The model under review builds one solid part; all positions refer to its coordinate system, in mm. A direction names the side the tool comes from. Round coordinates to 2 decimals unless told otherwise and drop trailing zeros. Order: outer loops, then holes, each group sorted by start corner. A loop starts at its lowest first (then second) coordinate and runs counter-clockwise, first axis right, second up. Notation, with made-up numbers: M -24,33 L 20,33 A35 ccw 20,72 Z; hole C 88.5,1.5 d5. An arc over 180 degrees is marked long. Answer as CSV lines item,"result". Start each with the question number.
from build123d import *

# Parameters (mm, degrees)
SKETCH1_R           = 1.525
SKETCH1_W           = 3
SKETCH1_H           = 19.5
BOSS_EXTRUDE1_DEPTH = 5
FILLET4_R           = 3
FILLET5_R           = 1
SKETCH4_R           = 3
CUT_EXTRUDE1_DEPTH  = 3
FILLET6_R           = 8
SKETCH6_R           = 19.727216355
CUT_EXTRUDE2_DEPTH  = 6
SKETCH9_R           = 9
CUT_EXTRUDE3_DEPTH  = 8.5
SKETCH11_W          = 2
SKETCH11_H          = 5
SKETCH11_W_2        = 10
SKETCH11_H_2        = 3
CUT_EXTRUDE4_DEPTH  = 6
FILLET7_R           = 1
SKETCH13_R          = 1.525
SKETCH13_W          = 3.25
SKETCH13_H          = 9
CUT_EXTRUDE5_DEPTH  = 6
FILLET8_R           = 1


with BuildPart() as part:
    # Sketch1 → Boss-Extrude1 (new body)
    with BuildSketch(Plane(origin=(0, 0, 0), x_dir=(1, 0, 0), z_dir=(0, 1, 0))):
        Polygon((-26.68337521, 71.16), (-26.68337521, 34), (-32.68337521, 28), (-20.1, 28), (-20.1, -28), (-32.68337521, -28), (-26.68337521, -34), (-26.68337521, -62.15662479), (-20, -68.84), (-20, -111.84), (20, -111.84), (20, -68.84), (26.68337521, -62.15662479), (26.68337521, -34), (32.68337521, -28), (25.1, -28), (25.1, -21), (45.1, -21), (45.1, 28), (32.68337521, 28), (26.68337521, 34), (26.68337521, 71.16), (16.68337521, 81.16), (-16.68337521, 81.16), align=None)
        with Locations(Location((-20.68337521, 71.16, 0), (0, 0, 270))):
            Circle(SKETCH1_R, mode=Mode.SUBTRACT)
        with Locations(Location((20.68337521, 71.16, 0), (0, 0, 270))):
            Circle(SKETCH1_R, mode=Mode.SUBTRACT)
        with Locations((1.4, 16.75)):
            Rectangle(SKETCH1_W, SKETCH1_H, mode=Mode.SUBTRACT)
        with Locations(Location((14.75, -40.84, 0), (0, 0, 270))):
            Circle(SKETCH1_R, mode=Mode.SUBTRACT)
        with Locations(Location((-14.75, -40.84, 0), (0, 0, 270))):
            Circle(SKETCH1_R, mode=Mode.SUBTRACT)
    extrude(amount=BOSS_EXTRUDE1_DEPTH)

    # Fillet4
    fillet4_edges = [part.edges().sort_by_distance(p)[0] for p in [
        (45.1, 2.5, -28),
    ]]
    fillet(fillet4_edges, radius=FILLET4_R)

    # Fillet5
    fillet5_edges = [part.edges().sort_by_distance(p)[0] for p in [
        (-0.1, 2.5, -26.5),
        (-0.1, 2.5, -7),
        (2.9, 2.5, -7),
        (2.9, 2.5, -26.5),
        (45.1, 2.5, 21),
        (25.1, 2.5, 21),
        (25.1, 2.5, 28),
        (32.68337521, 2.5, 28),
        (-32.68337521, 2.5, 28),
        (-20.1, 2.5, 28),
        (-20.1, 2.5, -28),
        (-32.68337521, 2.5, -28),
    ]]
    fillet(fillet5_edges, radius=FILLET5_R)

    # Sketch4 → Cut-Extrude1 (cut)
    with BuildSketch(Plane(origin=(0, 5, 0), x_dir=(1, 0, 0), z_dir=(0, 1, 0))):
        with Locations(Location((-20.68337521, 71.16, 0), (0, 0, 270))):
            Circle(SKETCH4_R)
        with Locations(Location((20.68337521, 71.16, 0), (0, 0, 270))):
            Circle(SKETCH4_R)
        with Locations(Location((-14.75, -40.84, 0), (0, 0, 270))):
            Circle(SKETCH4_R)
        with Locations(Location((14.75, -40.84, 0), (0, 0, 270))):
            Circle(SKETCH4_R)
    extrude(amount=-CUT_EXTRUDE1_DEPTH, mode=Mode.SUBTRACT)

    # Fillet6
    fillet6_edges = [part.edges().sort_by_distance(p)[0] for p in [
        (20, 2.5, 111.84),
        (-20, 2.5, 111.84),
    ]]
    fillet(fillet6_edges, radius=FILLET6_R)

    # Sketch6 → Cut-Extrude2 (cut)
    with BuildSketch(Plane(origin=(12.2, 0, 0), x_dir=(0, 0, -1), z_dir=(1, 0, 0))):
        with Locations((-83.11, -17)):
            Circle(SKETCH6_R)
    extrude(amount=-CUT_EXTRUDE2_DEPTH, mode=Mode.SUBTRACT)

    # Sketch9 → Cut-Extrude3 (cut)
    with BuildSketch(Plane(origin=(0, 0, -46.16), x_dir=(-1, 0, 0), z_dir=(0, 0, -1))):
        with Locations((0.16337521, -7.9)):
            Circle(SKETCH9_R)
    extrude(amount=-CUT_EXTRUDE3_DEPTH, mode=Mode.SUBTRACT)

    # Sketch11 → Cut-Extrude4 (cut)
    with BuildSketch(Plane(origin=(0, 5, 0), x_dir=(1, 0, 0), z_dir=(0, 1, 0))):
        with Locations((-19, -58.219322965)):
            Rectangle(SKETCH11_W, SKETCH11_H)
        with Locations((19, -58.219322965)):
            Rectangle(SKETCH11_W, SKETCH11_H)
        with Locations((0, -32.5)):
            Rectangle(SKETCH11_W_2, SKETCH11_H_2)
    extrude(amount=-CUT_EXTRUDE4_DEPTH, mode=Mode.SUBTRACT)

    # Fillet7
    fillet7_edges = [part.edges().sort_by_distance(p)[0] for p in [
        (-18, 2.5, 55.719322965),
        (-20, 2.5, 55.719322965),
        (-18, 2.5, 60.719322965),
        (-20, 2.5, 60.719322965),
        (20, 2.5, 60.719322965),
        (18, 2.5, 60.719322965),
        (18, 2.5, 55.719322965),
        (20, 2.5, 55.719322965),
        (5, 2.5, 31),
        (5, 2.5, 34),
        (-5, 2.5, 34),
        (-5, 2.5, 31),
    ]]
    fillet(fillet7_edges, radius=FILLET7_R - 0.0001)  # a hair under: the kernel refuses the full size

    # Sketch13 → Cut-Extrude5 (cut)
    with BuildSketch(Plane(origin=(0, 5, 0), x_dir=(1, 0, 0), z_dir=(0, 1, 0))):
        with Locations(Location((-6, 74.16, 0), (0, 0, 270))):
            Circle(SKETCH13_R)
        with Locations(Location((6, 74.16, 0), (0, 0, 270))):
            Circle(SKETCH13_R)
        with Locations((20.68337521, 57.226482401)):
            Rectangle(SKETCH13_W, SKETCH13_H)
    extrude(amount=-CUT_EXTRUDE5_DEPTH, mode=Mode.SUBTRACT)

    # Fillet8
    fillet8_edges = [part.edges().sort_by_distance(p)[0] for p in [
        (22.30837521, 2.5, -61.726482401),
        (22.30837521, 2.5, -52.726482401),
        (19.05837521, 2.5, -52.726482401),
        (19.05837521, 2.5, -61.726482401),
    ]]
    fillet(fillet8_edges, radius=FILLET8_R)


solid = part.part
Item 1: For pin 1 (1.4 mm diameter, centred on x = 20.5, y = 3.5, fed in from -Z); pin 2 (1 mm diameter, centred on y = 2.5, z = -35, fed in from +X); pin 3 (1.8 mm diameter, centred on x = 19.5, z = -72.5, fed in from +Y), all flat-tipped, find the tip position at first contact; note any pin that passes through.
Item 2: The part is to be moulded in two halves that separate along Z. For faces 1 (the flat face through (21, 2, -73)), 2 (the cylindrical face through (13.6, 3.52, 43.61)), 3 (the flat face through (23.29, 2.46, 65.55)), 4 (the flat face through (45.1, 2, -2)), say which applies: +Z half, -Z half, draft (parallel to the pull), parting line (faces both ways), or undercut.
Item 3: Tool access review of faces 5 (the flat face through (28, 2, 28)), 6 (the cylindrical face through (-0.2, 1.1, -42)), 7 (the flat face through (-26, 2, -28)), 8 (the flat face through (-26.683, 2, 48)): name each direction out of +Z, -Z, +X, -X, +Y, -Y from which nothing blocks a thin tool from reaching the whole face with its end or side.
Item 4: Wall thickness on probe 1 along X at (y, z) = (1, 40.84) (3 decimals); probe 2 along X at (y, z) = (3.7, 40.84); probe 3 along X at (y, z) = (3.5, -21.5): over which ranges is each line inside the solid? List them lowest first. Write a range as [from, to].
Item 5: Consider section A-A (z = -57.5). State the section outline as (x, y) points.
Item 6: Consider section B-B (z = 99). State the section outline as (x, y) points, and give its area (3 significant figures).
Reported:
1,pin 1,"stops at z = -78.04"
1,pin 2,"stops at x = 26.68"
1,pin 3,"stops at y = 2"
2,face 1,"undercut"
2,face 2,"undercut"
2,face 3,"+Z half"
2,face 4,"draft"
3,face 5,"+X, +Y, -Y"
3,face 6,"-Y"
3,face 7,"-X, +Y, -Y"
3,face 8,"+Z, -X, +Y, -Y"
4,probe 1,"x = [-26.683, -16.275], [-13.225, 13.225], [16.275, 26.683]"
4,probe 2,"x = [-26.68, -17.75], [-11.75, 11.75], [17.75, 26.68]"
4,probe 3,"x = [-20.1, -0.1], [2.9, 45.1]"
5,outline,"M -26.68,0 L 19.06,0 L 19.06,5 L -26.68,5 Z; M 22.31,0 L 26.68,0 L 26.68,5 L 22.31,5 Z"
6,outline,"M -20,0 L 20,0 L 20,5 L -20,5 Z"
6,area,"200 mm²"
